Source: CAD feature listing. Evaluate the final solid. Frame: model axes, mm. Round coordinates to 2 decimals unless told otherwise and drop trailing zeros. Write each loop counter-clockwise with the first axis right and the second up, starting at its lowest first coordinate (ties: lowest second). Pieces come first, ordered by that corner, then holes. Notation, with made-up numbers: (7, -10.5) -> (22, -10.5) arc R15 cw to (22, 9.5) -> close; hole circle Ø2 at (65.5, 56.25). An arc over 180 degrees is marked (long way). Put each result on its own line as item: value.
```python
from build123d import *

# Parameters (mm, degrees)
F0_W     = 25
F0_H     = 25
F0_R     = 1.65
F1_DEPTH = 20
F2_DEPTH = 25
F3_R     = 1.4
F4_DEPTH = 12.5
F6_D     = 3


with BuildPart() as f1:
    # F0 (on Top) → F1 (new body)
    with BuildSketch(Plane.XY):
        Rectangle(F0_W, F0_H)
        with Locations((0, -4)):
            Circle(F0_R, mode=Mode.SUBTRACT)
        with Locations((0, 4)):
            Circle(F0_R, mode=Mode.SUBTRACT)
    extrude(amount=F1_DEPTH)

    # F2 (add): a face of the model
    f2_faces = [f1.faces().sort_by_distance(p)[0] for p in [
        (-12.5, 0, 10),
    ]]
    extrude(f2_faces, amount=F2_DEPTH)

    # F3 (on Front) → F4 (cut, symmetric)
    with BuildSketch(Plane.XZ):
        with BuildLine():
            add(Edge.make_bspline(
                [(-37.5, 12), (-33.778607057, 12.0509013714), (-25.1001296566, 12.3187041592), (-15.8211888541, 11.1248698681), (-12.5, 0)],
                knots=[0, 0, 0, 0, 0.44474528, 1, 1, 1, 1], degree=3))
            Line((-37.5, 12), (-37.5, 0))
            Line((-37.5, 0), (-12.5, 0))
        make_face()
        with Locations((-34, 19.8526792228)):
            Circle(F3_R)
        with Locations((-28, 19.8505632579)):
            Circle(F3_R)
    extrude(amount=F4_DEPTH, both=True, mode=Mode.SUBTRACT)

    # F6 (through all)
    with Locations(Plane(origin=(0, 0, 0), x_dir=(1, 0, 0), z_dir=(0, 0, -1))):
        with Locations((-31, 5), (-31, -5)):
            Hole(F6_D / 2)


solid = f1.part
```
Q1. Draft query along X for faces 1 (the flat face through (-7, 0, 20)), 2 (the flat face through (12.5, 0, 10)), 3 (the cylindrical face through (-29.5, 4.93, 16.09)). Return one class per face: +X half, -X half, draft (parallel to the pull), parting line (faces both ways), or undercut.
Ans:
face 1: draft
face 2: +X half
face 3: undercut
Q2. Cut plane B-B on z = 14. Output: boundary loops of the cut face in (x, y), and give its area (3 significant figures).
Ans:
outline: (-37.5, -12.5) -> (12.5, -12.5) -> (12.5, 12.5) -> (-37.5, 12.5) -> close; hole circle Ø3 at (-31, -5); hole circle Ø3 at (-31, 5); hole circle Ø3.3 at (0, -4); hole circle Ø3.3 at (0, 4)
area: 1,220 mm^2
Q3. Material intervals for line 1 (Y direction, x = 0, z = 6.75); line 2 (Y direction, x = -31, z = 17.75); line 3 (X direction, y = -5, z = 18), sorted ascending. Write a range as [from, to].
Ans:
line 1: y = [-12.5, -5.65], [-2.35, 2.35], [5.65, 12.5]
line 2: y = [-12.5, -6.5], [-3.5, 3.5], [6.5, 12.5]
line 3: x = [-37.5, -32.5], [-29.5, -1.31], [1.31, 12.5]
Q4. Cut plane C-C on y = -4. Give the number of separate pieces and of enclosed holes in the cut face, and give its area (3 significant figures).
Ans:
separate pieces: 3
enclosed holes: 0
area: 648 mm^2
Q5. Cut plane A-A on x = 0. Output: boundary loops of the cut face in (y, z).
Ans:
outline: (-12.5, 0) -> (-5.65, 0) -> (-5.65, 20) -> (-12.5, 20) -> close; (-2.35, 0) -> (2.35, 0) -> (2.35, 20) -> (-2.35, 20) -> close; (5.65, 0) -> (12.5, 0) -> (12.5, 20) -> (5.65, 20) -> close
Q6. Pin query (flat end, axial travel): pin 1 (5 mm diameter, centred on x = -27, y = -6.5, fed in from +Z); pin 2 (1.8 mm diameter, centred on x = -31, y = 5, fed in from +Z). Return the tip coordinate at first contact, or that it passes through.
Ans:
pin 1: stops at z = 20
pin 2: passes through
